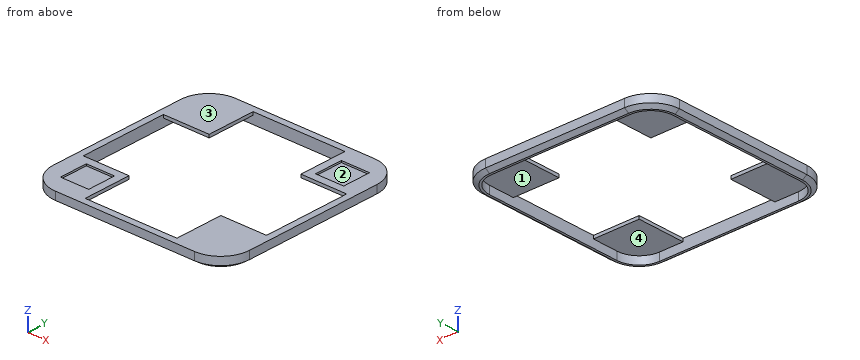
Autodesk Inventor part; units mm, degrees
ref_plane "YZ Plane" through (0, 0, 0) normal (1, 0, 0) x (0, 1, 0)
ref_plane "XZ Plane" through (0, 0, 0) normal (0, 1, 0) x (-1, 0, 0)
ref_plane "XY Plane" through (0, 0, 0) normal (0, 0, 1) x (1, 0, 0)
sketch "Skizze1" plane through (0, 0, 0) normal (0, 0, 1) x (1, 0, 0)
  line L0 (32.9869, 99.2902) -> (32.9869, 40.1902) construction
  arc A0 (22.9869, 30.1902) -> (32.9869, 40.1902) centre (22.9869, 40.1902) ccw construction
  line L1 (22.9869, 30.1902) -> (-36.1131, 30.1902) construction
  arc A1 (-46.1131, 40.1902) -> (-36.1131, 30.1902) centre (-36.1131, 40.1902) ccw construction
  line L2 (-46.1131, 40.1902) -> (-46.1131, 99.2902) construction
  arc A2 (-36.1131, 109.2902) -> (-46.1131, 99.2902) centre (-36.1131, 99.2902) ccw construction
  line L3 (-36.1131, 109.2902) -> (22.9869, 109.2902) construction
  arc A3 (32.9869, 99.2902) -> (22.9869, 109.2902) centre (22.9869, 99.2902) ccw construction
  arc A4 (-38.6131, 111.7902) -> (-48.6131, 101.7902) centre (-38.6131, 101.7902) ccw construction
  line L4 (-48.6131, 101.7902) -> (-48.6131, 37.6902) construction
  arc A5 (-48.6131, 37.6902) -> (-38.6131, 27.6902) centre (-38.6131, 37.6902) ccw construction
  line L5 (-38.6131, 27.6902) -> (25.4869, 27.6902) construction
  arc A6 (25.4869, 27.6902) -> (35.4869, 37.6902) centre (25.4869, 37.6902) ccw construction
  line L6 (35.4869, 37.6902) -> (35.4869, 101.7902) construction
  arc A7 (35.4869, 101.7902) -> (25.4869, 111.7902) centre (25.4869, 101.7902) ccw construction
  line L7 (25.4869, 111.7902) -> (-38.6131, 111.7902) construction
  arc A8 (-38.6131, 111.9702) -> (-48.7931, 101.7902) centre (-38.6131, 101.7902) ccw
  line L8 (-48.7931, 101.7902) -> (-48.7931, 37.6902)
  arc A9 (-48.7931, 37.6902) -> (-38.6131, 27.5102) centre (-38.6131, 37.6902) ccw
  line L9 (-38.6131, 27.5102) -> (25.4869, 27.5102)
  arc A10 (25.4869, 27.5102) -> (35.6669, 37.6902) centre (25.4869, 37.6902) ccw
  line L10 (35.6669, 37.6902) -> (35.6669, 101.7902)
  arc A11 (35.6669, 101.7902) -> (25.4869, 111.9702) centre (25.4869, 101.7902) ccw
  line L11 (25.4869, 111.9702) -> (-38.6131, 111.9702)
  arc A12 (-38.6131, 114.9702) -> (-51.7931, 101.7902) centre (-38.6131, 101.7902) ccw
  line L12 (-38.6131, 114.9702) -> (25.4869, 114.9702)
  arc A13 (38.6669, 101.7902) -> (25.4869, 114.9702) centre (25.4869, 101.7902) ccw
  line L13 (38.6669, 101.7902) -> (38.6669, 37.6902)
  arc A14 (25.4869, 24.5102) -> (38.6669, 37.6902) centre (25.4869, 37.6902) ccw
  line L14 (25.4869, 24.5102) -> (-38.6131, 24.5102)
  arc A15 (-51.7931, 37.6902) -> (-38.6131, 24.5102) centre (-38.6131, 37.6902) ccw
  line L15 (-51.7931, 37.6902) -> (-51.7931, 101.7902)
  line L16 (12.5869, 111.9702) -> (12.5869, 87.8902)
  line L17 (12.5869, 87.8902) -> (35.6669, 87.8902)
  circle A16 centre (24.5869, 99.8902) radius 5.075 construction
  circle A17 centre (-37.7131, 39.5902) radius 5.075 construction
  line L18 (-48.7931, 51.5902) -> (-25.7131, 51.5902)
  line L19 (-25.7131, 51.5902) -> (-25.7131, 27.5102)
  point P0 (0, 0)
  dimension "d0" = 0.18
  dimension "d1" = 3
  dimension "d2" = 12
  dimension "d3" = 12
  dimension "d4" = 12
  dimension "d5" = 12
extrude "Extrusion1" add sketch "Skizze1" along normal blind 5
chamfer "Fase1" distance 2 angle 35 8 edges at (34.8066, 111.1099, 0) (38.6669, 69.7402, 0) (34.8066, 28.3705, 0) (-6.5631, 24.5102, 0) (-47.9328, 28.3705, 0) (-51.7931, 69.7402, 0) (-47.9328, 111.1099, 0) (-6.5631, 114.9702, 0) measured on face at (-12.9464, 25.5102, 0)
sketch "Skizze2" plane through (0, 0, 5) normal (0, 0, 1) x (1, 0, 0)
  circle A0 centre (-37.7131, 39.5902) radius 5.075 construction
  circle A1 centre (24.5869, 99.8902) radius 5.075 construction
  line L0 (-48.7931, 37.6902) -> (-48.7931, 101.7902)
  line L1 (-48.7931, 49.5902) -> (-27.7131, 49.5902)
  line L2 (-27.7131, 49.5902) -> (-27.7131, 27.5102)
  line L3 (-38.6131, 27.5102) -> (25.4869, 27.5102)
  arc A2 (-48.7931, 37.6902) -> (-38.6131, 27.5102) centre (-38.6131, 37.6902) ccw
  line L4 (35.6669, 101.7902) -> (35.6669, 37.6902)
  arc A3 (35.6669, 101.7902) -> (25.4869, 111.9702) centre (25.4869, 101.7902) ccw
  line L5 (-38.6131, 111.9702) -> (25.4869, 111.9702)
  line L6 (25.4869, 111.9702) -> (-38.6131, 111.9702)
  line L7 (14.5869, 111.9702) -> (14.5869, 89.8902)
  line L8 (14.5869, 89.8902) -> (35.6669, 89.8902)
  arc A4 (-38.6131, 111.9702) -> (-48.7931, 101.7902) centre (-38.6131, 101.7902) ccw
  arc A5 (25.4869, 27.5102) -> (35.6669, 37.6902) centre (25.4869, 37.6902) ccw
  line L9 (14.5869, 27.5102) -> (14.5869, 49.5902)
  line L10 (14.5869, 49.5902) -> (35.6669, 49.5902)
  line L11 (35.6669, 37.6902) -> (35.6669, 101.7902)
  line L12 (-48.7931, 89.8902) -> (-27.7131, 89.8902)
  line L13 (-27.7131, 89.8902) -> (-27.7131, 111.9702)
  point P0 (0, 0)
  dimension "d11" = 10
  dimension "d12" = 10
  dimension "d13" = 10
  dimension "d14" = 10
extrude "Extrusion2" add sketch "Skizze2" against normal blind 1.4 contours L0 L1 L2 L3 A2 | L0 A4 L5 L13 L12 | L9 L10 L4 A5 L3 | L5 A3 L4 L8 L7
sketch "Skizze3" plane through (0, 0, 5) normal (0, 0, 1) x (1, 0, 0)
  circle A0 centre (-37.7131, 39.5902) radius 5.075 construction
  circle A1 centre (24.5869, 99.8902) radius 4.075 construction
  line L0 (18.0869, 93.3902) -> (31.0869, 93.3902)
  line L1 (31.0869, 93.3902) -> (31.0869, 106.3902)
  line L2 (31.0869, 106.3902) -> (18.0869, 106.3902)
  line L3 (18.0869, 106.3902) -> (18.0869, 93.3902)
  line L4 (18.0869, 93.3902) -> (31.0869, 106.3902) construction
  line L5 (31.0869, 93.3902) -> (18.0869, 106.3902) construction
  line L6 (-44.2131, 33.0902) -> (-31.2131, 33.0902)
  line L7 (-31.2131, 33.0902) -> (-31.2131, 46.0902)
  line L8 (-31.2131, 46.0902) -> (-44.2131, 46.0902)
  line L9 (-44.2131, 46.0902) -> (-44.2131, 33.0902)
  line L10 (-44.2131, 33.0902) -> (-31.2131, 46.0902) construction
  line L11 (-31.2131, 33.0902) -> (-44.2131, 46.0902) construction
  point P0 (0, 0)
  dimension "d17" = 13
  dimension "d18" = 13
  dimension "d19" = 13
  dimension "d20" = 13
extrude "Extrusion3" cut sketch "Skizze3" against normal blind 0.8
equation "\"d2\" = d3"
equation "\"d4\" = d3"
equation "\"d5\" = d4"
properties part number "Wandhalterung"
The listing builds one solid part. Answer for the finished solid, in the listing's coordinates (mm). Face numbers are marked on the shaded views. A direction names the side the tool comes from. Round coordinates to 2 decimals unless told otherwise and drop trailing zeros. Loops run counter-clockwise (first coordinate to the right, second up) from the corner with the lowest first, then second, coordinate; pieces in that order, holes last. Notation, with made-up numbers: (79, 27.25) - (134, 27.25) arc R21 cw to (134, 39.25) - close; hole circle Ø4 at (86.25, 79). An arc over 180 degrees is marked (long way). Use one line per item in the form item = value. Start each with the question number.
1. A tool of negligible diameter and unlimited length cuts with its end or side. For the marked faces 1 and 2, from which of +Z, -Z, +X, -X, +Y, -Y can it reach the whole face along a straight path? Write none if from no direction.
2. Consider line 1 (Y direction, x = 25, z = 4.45); line 2 (Y direction, x = 9, z = 2.6); line 3 (X direction, y = 83.5, z = 2.7). Determine where each line is inside the solid, lowest interval first. Write a range as [from, to].
3. The part is cut by section B-B on y = 65. Determine the outline of the cut face in (x, z), then the cut area to 3 significant figures.
4. The part is cut by section C-C on x = 23.5. Determine the outline of the cut face in (y, z).
5. For a pull along Y with two mould halves and no side action, classify the marked faces 3 and 4 as pulls with the +Y half, pulls with the -Y half, needs draft (parallel to the pull), parting line crosses it, or undercut.
6. The part is cut by section A-A on x = -3. Determine the outline of the cut face in (y, z).
7. Given pin 1 Ø1.1 at (x, z) = (27.5, 4.5) entering from +Y; pin 2 Ø3 at (x, y) = (-32.5, 36.5) entering from -Z; pin 3 Ø4 at (x, y) = (-38, 40.5) entering from +Z, each flat-ended and moving along its own axis, determine where each tip first touches the part or whether it passes through.
Geometry check:
q1.face_1 = -Z
q1.face_2 = +Z
q2.line_1 = [24.51, 49.59], [89.89, 93.39], [106.39, 114.97]
q2.line_2 = [24.51, 27.51], [111.97, 114.97]
q2.line_3 = [-51.79, -48.79], [35.67, 38.67]
q3.outline = (-51.79, 1.4) - (-49.79, 0) - (-48.79, 0) - (-48.79, 5) - (-51.79, 5) - close; (35.67, 0) - (36.67, 0) - (38.67, 1.4) - (38.67, 5) - (35.67, 5) - close
q3.area = 27.2 mm^2
q4.outline = (24.51, 1.4) - (26.51, 0) - (27.51, 0) - (27.51, 3.6) - (49.59, 3.6) - (49.59, 5) - (24.51, 5) - close; (89.89, 3.6) - (111.97, 3.6) - (111.97, 0) - (112.97, 0) - (114.97, 1.4) - (114.97, 5) - (106.39, 5) - (106.39, 4.2) - (93.39, 4.2) - (93.39, 5) - (89.89, 5) - close
q5.face_3 = needs draft
q5.face_4 = undercut
q6.outline = (24.51, 1.4) - (26.51, 0) - (27.51, 0) - (27.51, 5) - (24.51, 5) - close; (111.97, 0) - (112.97, 0) - (114.97, 1.4) - (114.97, 5) - (111.97, 5) - close
q7.pin_1 = 114.89
q7.pin_2 = 3.6
q7.pin_3 = 4.2
